Here's how the part is built. I have some questions about the finished solid (model axes, mm). Face numbers are marked on the shaded views. A direction names the side the tool comes from. Round coordinates to 2 decimals unless told otherwise and drop trailing zeros. Write each loop counter-clockwise with the first axis right and the second up, starting at its lowest first coordinate (ties: lowest second). Pieces come first, ordered by that corner, then holes. Notation, with made-up numbers: (54.25, 39) - (72.25, 39) arc R32 cw to (72.25, 78) - close; hole circle Ø8 at (-32, -5). An arc over 180 degrees is marked (long way). One line per question, with ' | ' between items. Start each with the question number.
(1) For the marked faces 5 and 6, which set-ups out of +Z, -Z, +X, -X, +Y, -Y let a thin tool reach every point of the face, with its end or its side?
(2) Imagine slicing it at D-D (z = 25). Write out the boundary of the cut face in (x, y), plus the area to 3 significant figures.
(3) Will these pins go through, and if not, where does the flat tip stop? pin 1 (6 mm diameter, centred on x = 4.5, z = 6, fed in from +Y); pin 2 (14.5 mm diameter, centred on x = -34, z = -20, fed in from +Y).
(4) Imagine slicing it at C-C (z = -20). Write out the boundary of the cut face in (x, y), plus the area to 3 significant figures.
(5) Imagine slicing it at B-B (y = 19.5). Write out the boundary of the cut face in (x, z).
(6) If I drill on L1, parallel to X at y = 19.25, z = 5; L2, parallel to Z at x = -16.5, y = 4.5; L3, parallel to Z at x = -10, y = 0.7, over which ranges is the centre line in solid material (lowest first)?
(7) Thinking about a two-plate mould opening in X: for the marked faces 1, 2, 3 and 4, which applies, pulls with the +X half, pulls with the -X half, needs draft (parallel to the pull), parting line crosses it, or undercut?
(8) Imagine slicing it at A-A (x = -10). Write out the boundary of the cut face in (y, z).
from build123d import *

# Parameters (mm, degrees)
ESQUISSE1_W             = 100
ESQUISSE1_H             = 80
BOSS_EXTRU_1_DEPTH      = 2
ESQUISSE2_W             = 100
ESQUISSE2_H             = 80
ESQUISSE2_W_2           = 96
ESQUISSE2_H_2           = 76
BOSS_EXTRU_2_DEPTH      = 20
ESQUISSE5_W             = 100
ESQUISSE5_H             = 80
ESQUISSE5_W_2           = 98.2
ESQUISSE5_H_2           = 78.2
BOSS_EXTRU_3_DEPTH      = 2
ESQUISSE6_W             = 18
ESQUISSE6_H             = 2
ENL_V_MAT_EXTRU_3_DEPTH = 10
CONG_1_R                = 1
ESQUISSE7_R             = 8
ENL_V_MAT_EXTRU_4_DEPTH = 10


with BuildPart() as part:
    # Esquisse1 → Boss.-Extru.1 (new body)
    with BuildSketch(Plane(origin=(0, 0, 0), x_dir=(1, 0, 0), z_dir=(0, 1, 0))):
        Rectangle(ESQUISSE1_W, ESQUISSE1_H)
    extrude(amount=BOSS_EXTRU_1_DEPTH)

    # Esquisse2 → Boss.-Extru.2 (add)
    with BuildSketch(Plane(origin=(0, 2, 0), x_dir=(1, 0, 0), z_dir=(0, 1, 0))):
        Rectangle(ESQUISSE2_W, ESQUISSE2_H)
        Rectangle(ESQUISSE2_W_2, ESQUISSE2_H_2, mode=Mode.SUBTRACT)
    extrude(amount=BOSS_EXTRU_2_DEPTH)

    # Esquisse5 → Boss.-Extru.3 (add)
    with BuildSketch(Plane(origin=(0, 22, 0), x_dir=(1, 0, 0), z_dir=(0, 1, 0))):
        Rectangle(ESQUISSE5_W, ESQUISSE5_H)
        Rectangle(ESQUISSE5_W_2, ESQUISSE5_H_2, mode=Mode.SUBTRACT)
    extrude(amount=BOSS_EXTRU_3_DEPTH)

    # Esquisse6 → Enlèv. mat.-Extru.3 (cut)
    with BuildSketch(Plane(origin=(0, 0, -40), x_dir=(-1, 0, 0), z_dir=(0, 0, -1))):
        with Locations((30, 23)):
            Rectangle(ESQUISSE6_W, ESQUISSE6_H)
    extrude(amount=-ENL_V_MAT_EXTRU_3_DEPTH, mode=Mode.SUBTRACT)

    # Congé1
    cong_1_edges = [part.edges().sort_by_distance(p)[0] for p in [
        (-39, 22, -39.55),
        (-21, 22, -39.55),
    ]]
    fillet(cong_1_edges, radius=CONG_1_R)

    # Esquisse7 → Enlèv. mat.-Extru.4 (cut)
    with BuildSketch(Plane.XZ):
        with Locations((-34, -20)):
            Circle(ESQUISSE7_R)
        with Locations((-10, -20)):
            Circle(ESQUISSE7_R)
    extrude(amount=-ENL_V_MAT_EXTRU_4_DEPTH, mode=Mode.SUBTRACT)


solid = part.part
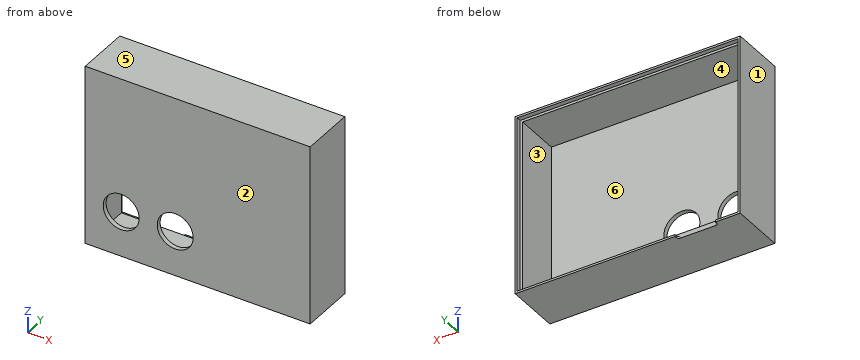
Check sheet entries:
1) face 5: +Z, +X, -X, +Y, -Y | face 6: +Y
2) outline: (-50, 0) - (50, 0) - (50, 24) - (49.1, 24) - (49.1, 22) - (48, 22) - (48, 2) - (-48, 2) - (-48, 22) - (-49.1, 22) - (-49.1, 24) - (-50, 24) - close | area: 284 mm^2
3) pin 1: y = 2 | pin 2: through
4) outline: (-50, 0) - (-42, 0) - (-42, 2) - (-48, 2) - (-48, 22) - (-49.1, 22) - (-49.1, 24) - (-50, 24) - close; (-26, 0) - (-18, 0) - (-18, 2) - (-26, 2) - close; (-2, 0) - (50, 0) - (50, 24) - (49.1, 24) - (49.1, 22) - (48, 22) - (48, 2) - (-2, 2) - close | area: 220 mm^2
5) outline: (-50, -40) - (50, -40) - (50, 40) - (-50, 40) - close; hole (-48, -38) - (48, -38) - (48, 38) - (-48, 38) - close
6) L1: -50 to -48, 48 to 50 | L2: -40 to -38, 38 to 40 | L3: -40 to -28, -12 to 40
7) face 1: pulls with the -X half | face 2: needs draft | face 3: undercut | face 4: undercut
8) outline: (0, -40) - (24, -40) - (24, -39.1) - (22, -39.1) - (22, -38) - (2, -38) - (2, -28) - (0, -28) - close; (0, -12) - (2, -12) - (2, 38) - (22, 38) - (22, 39.1) - (24, 39.1) - (24, 40) - (0, 40) - close
